For this review, take the finished solid that the model builds, in its own axes (mm). A direction names the side the tool comes from. Give positions to 0.01 mm unless a question says otherwise; leave off trailing zeros. Loops run counter-clockwise (first coordinate to the right, second up) from the corner with the lowest first, then second, coordinate; pieces in that order, holes last. Notation, with made-up numbers: (-11, -10.5) - (-7, -10.5) arc R25 cw to (-7, 3.5) - close; hole circle Ø2 at (33.5, -35). An arc over 180 degrees is marked (long way). Answer in a Markdown table with one row per item.
Autodesk Inventor part; units mm, degrees
ref_plane "YZ Plane" through (0, 0, 0) normal (1, 0, 0) x (0, 1, 0)
ref_plane "XZ Plane" through (0, 0, 0) normal (0, 1, 0) x (-1, 0, 0)
ref_plane "XY Plane" through (0, 0, 0) normal (0, 0, 1) x (1, 0, 0)
sketch "Sketch1" plane through (0, 0, 0) normal (0, 0, 1) x (1, 0, 0)
  line L0 (0, 0) -> (65, 0)
  line L1 (65, 0) -> (65, 3)
  line L2 (65, 3) -> (0, 3)
  line L3 (0, 3) -> (0, 0)
  dimension "d0" = 65
  dimension "d1" = 6
revolve "Revolution1" add sketch "Sketch1" angle 360 about axis through (0, 0, 0) along (1, 0, 0)
thread "Thread1"
chamfer "Chamfer1" distance 1 angle 45 2 edges at (0, -3, 0) (65, -3, 0)
sketch "Sketch2" plane through (0, 0, 0) normal (0, 0, 1) x (1, 0, 0)
  line L0 (1, 3) -> (64, 3)
  line L1 (65, 3) -> (55, 3)
  line L2 (55, 3) -> (55, 2)
  line L3 (55, 2) -> (65, 2)
  line L4 (65, 2) -> (65, 3)
  line L5 (65, -3) -> (65, 3)
  line L6 (65, -3) -> (55, -3)
  line L7 (55, -3) -> (55, -2)
  line L8 (55, -2) -> (65, -2)
  line L9 (65, -2) -> (65, -3)
  point P0 (0, 0)
  point P1 (55, 3)
  dimension "d8" = 4
  dimension "d15" = 10
extrude "Extrusion1" cut sketch "Sketch2" along normal through all both and the other way through all
sketch "Sketch3" plane through (55, -2, -2.2361) normal (0, -1, 0) x (1, 0, 0)
  circle A0 centre (7, 2.2361) radius 2
  line L0 (10, 2.2361) -> (10, 0.2361)
  point P0 (-55, 2.2361)
  dimension "d11" = 4
  dimension "d14" = 3
extrude "Extrusion2" cut sketch "Sketch3" against normal through all
properties part number "M6x1_THREADED_ROD" material "Steel, Carbon"
1. Wall thickness on line 1 (X direction, y = -1, z = 0.05); line 2 (Z direction, x = 61, y = -0.2); line 3 (Z direction, x = 62, y = 0.6): over which ranges is each line inside the solid? List them lowest first. Write a range as [from, to].
Values:
| item | result |
|---|---|
| line 1 | x = [0, 60], [64, 65] |
| line 2 | z = [-2.99, -1.73], [1.73, 2.99] |
| line 3 | z = [-2.94, -2], [2, 2.94] |
2. We need section A-A, the plane x = 62. Give the boundary of the cut face in (y, z), and give its area (3 significant figures).
Values:
| item | result |
|---|---|
| outline | (-2, -2.24) arc R3 ccw to (2, -2.24) - (2, -2) - (-2, -2) - close; (-2, 2) - (2, 2) - (2, 2.24) arc R3 ccw to (-2, 2.24) - close |
| area | 6.08 mm^2 |
3. Clearance check with flat-ended pins moving along their axes: pin 1 (0.8 mm diameter, centred on y = -2.5, z = -1, fed in from +X); pin 2 (1 mm diameter, centred on x = 15, y = 2.5, fed in from -Z); pin 3 (2 mm diameter, centred on x = 20.5, y = -1.5, fed in from +Z). State where each tip first meets the part, or that it passes through.
Values:
| item | result |
|---|---|
| pin 1 | stops at x = 55 |
| pin 2 | stops at z = -2.24 |
| pin 3 | stops at z = 2.96 |
4. We need section C-C, the plane x = 46. Give the boundary of the cut face in (y, z), and give its area (3 significant figures).
Values:
| item | result |
|---|---|
| outline | circle Ø6 at (0, 0) |
| area | 28.3 mm^2 |
5. We need section B-B, the plane y = 0. Give the boundary of the cut face in (x, z), and give its area (3 significant figures).
Values:
| item | result |
|---|---|
| outline | (0, -2) - (1, -3) - (64, -3) - (65, -2) - (65, 2) - (64, 3) - (1, 3) - (0, 2) - close; hole circle Ø4 at (62, 0) |
| area | 375 mm^2 |
6. For faces 1 (the face through (65, 0, 0)), 2 (the face through (55, 2.4, 0)), 3 (the face through (55, -2.4, 0)), list the 3-axis set-ups (+Z, -Z, +X, -X, +Y, -Y) from which the entire face can be reached by the end or side of a thin tool; tool diameter is ignored.
Values:
| item | result |
|---|---|
| face 1 | +Z, -Z, +X, +Y, -Y |
| face 2 | +Z, -Z, +X, +Y |
| face 3 | +Z, -Z, +X, -Y |
7. Mouldability with a two-part tool opening along Z and no side actions: class faces 4 (the face through (60, 0, 0)), 5 (the face through (59, -2, 0)), 6 (the face through (64.7, -0.1, 2.3)) as released by +Z, released by -Z, zero draft, split by the parting line, or undercut.
Values:
| item | result |
|---|---|
| face 4 | undercut |
| face 5 | zero draft |
| face 6 | released by +Z |
